Could you check a few things on this model? Use its own coordinates, in mm. A direction names the side the tool comes from. Round coordinates to 2 decimals unless told otherwise and drop trailing zeros. Loops run counter-clockwise (first coordinate to the right, second up) from the corner with the lowest first, then second, coordinate; pieces in that order, holes last. Notation, with made-up numbers: (0.5, 79) -> (39.5, 79) arc R17 ccw to (39.5, 87) -> close; hole circle Ø9 at (-31.5, 66). An arc over 180 degrees is marked (long way). One line per item, written item: value.
from build123d import *

# Parameters (mm, degrees)
BODY_DEPTH                     = 5
BODY_DEPTH_BACK                = 5
SKETCH2_R                      = 0.85
F_1_7MM_THRU_SCREW_HOLES_DEPTH = 15
SCREWHEAD_RELIEF_DEPTH         = 0.5
SKETCH4_R                      = 1.05
F_1_P_PORT_DEPTH               = 5
SKETCH5_R                      = 1.05
F_2_B_PORT_DEPTH               = 5
SKETCH6_R                      = 1.05
F_3_R2_PORT_DEPTH              = 5
SKETCH7_R                      = 1.05
F_4_A_PORT_DEPTH               = 5
SKETCH8_R                      = 1.05
F_5_R1_PORT_DEPTH              = 5
EXTRUDE3_DEPTH                 = 1
FILLET1_R                      = 0.5
SKETCH10_R                     = 0.75
WIRES_2_DEPTH                  = 5


with BuildPart() as part:
    # Sketch1 → Body (new body, two sides)
    with BuildSketch(Plane(origin=(0, 0, 0), x_dir=(0, 0, -1), z_dir=(1, 0, 0))) as body_sk:
        Polygon((0, 0), (-58.6, 0), (-58.6, -14), (-22.5, -14), (-22.5, -19.6), (-4, -19.6), (-4, -14), (0, -14), align=None)
    extrude(amount=BODY_DEPTH)
    extrude(body_sk.sketch, amount=-BODY_DEPTH_BACK)

    # Sketch2 → 1.7mm Thru Screw Holes (cut, through all)
    with BuildSketch(Plane.XZ.offset(14)):
        with Locations(Location((-3.7, 41.9, 0), (0, 0, 270))):  # turned: the seam where the file's is
            Circle(SKETCH2_R)
        with Locations(Location((3.7, 45.5, 0), (0, 0, 270))):  # turned: the seam where the file's is
            Circle(SKETCH2_R)
    extrude(amount=-F_1_7MM_THRU_SCREW_HOLES_DEPTH, mode=Mode.SUBTRACT)

    # Sketch3 → Screwhead Relief (cut)
    with BuildSketch(Plane.XZ.offset(14)):
        with BuildLine():
            Line((-3.7, 43.7), (-5, 43.7))
            Line((-5, 43.7), (-5, 40.1))
            Line((-5, 40.1), (-3.7, 40.1))
            ThreePointArc((-3.7, 40.1), (-1.9, 41.9), (-3.7, 43.7))
        make_face()
        with BuildLine():
            Line((3.7, 47.3), (5, 47.3))
            Line((5, 47.3), (5, 43.7))
            Line((5, 43.7), (3.7, 43.7))
            ThreePointArc((3.7, 43.7), (1.9, 45.5), (3.7, 47.3))
        make_face()
    extrude(amount=-SCREWHEAD_RELIEF_DEPTH, mode=Mode.SUBTRACT)

    # Sketch4 → 1 P _port (cut)
    with BuildSketch(Plane(origin=(0, 0, 0), x_dir=(-1, 0, 0), z_dir=(0, 1, 0))):
        with Locations(Location((0, 43.7, 0), (0, 0, 90))):  # turned: the seam where the file's is
            Circle(SKETCH4_R)
    extrude(amount=-F_1_P_PORT_DEPTH, mode=Mode.SUBTRACT)

    # Sketch5 → 2 B _port (cut)
    with BuildSketch(Plane(origin=(0, 0, 0), x_dir=(-1, 0, 0), z_dir=(0, 1, 0))):
        with Locations(Location((2.5, 47.3, 0), (0, 0, 90))):  # turned: the seam where the file's is
            Circle(SKETCH5_R)
    extrude(amount=-F_2_B_PORT_DEPTH, mode=Mode.SUBTRACT)

    # Sketch6 → 3 R2 _port (cut)
    with BuildSketch(Plane(origin=(0, 0, 0), x_dir=(-1, 0, 0), z_dir=(0, 1, 0))):
        with Locations(Location((0, 50.9, 0), (0, 0, 90))):  # turned: the seam where the file's is
            Circle(SKETCH6_R)
    extrude(amount=-F_3_R2_PORT_DEPTH, mode=Mode.SUBTRACT)

    # Sketch7 → 4 A _port (cut)
    with BuildSketch(Plane(origin=(0, 0, 0), x_dir=(-1, 0, 0), z_dir=(0, 1, 0))):
        with Locations(Location((-2.5, 40.1, 0), (0, 0, 90))):  # turned: the seam where the file's is
            Circle(SKETCH7_R)
    extrude(amount=-F_4_A_PORT_DEPTH, mode=Mode.SUBTRACT)

    # Sketch8 → 5 R1 _port (cut)
    with BuildSketch(Plane(origin=(0, 0, 0), x_dir=(-1, 0, 0), z_dir=(0, 1, 0))):
        with Locations(Location((0, 36.5, 0), (0, 0, 90))):  # turned: the seam where the file's is
            Circle(SKETCH8_R)
    extrude(amount=-F_5_R1_PORT_DEPTH, mode=Mode.SUBTRACT)

    # Sketch9 → Extrude3 (add)
    with BuildSketch(Plane.XZ.offset(19.6)):
        with BuildLine():
            Line((-1.5, 9.5), (1.5, 9.5))
            ThreePointArc((1.5, 9.5), (3.5, 7.5), (1.5, 5.5))
            Line((1.5, 5.5), (-1.5, 5.5))
            ThreePointArc((-1.5, 5.5), (-3.5, 7.5), (-1.5, 9.5))
        make_face()
    extrude(amount=EXTRUDE3_DEPTH)

    # Fillet1
    fillet1_edges = [part.edges().sort_by_distance(p)[0] for p in [
        (-3.5, -20.6, 7.5),
        (0, -20.6, 5.5),
        (3.5, -20.6, 7.5),
        (0, -20.6, 9.5),
    ]]
    fillet(fillet1_edges, radius=FILLET1_R)

    # Sketch10 → Wires 2 (add)
    with BuildSketch(Plane.XZ.offset(20.6)):
        with Locations(Location((-1.5, 7.5, 0), (0, 0, 270))):  # turned: the seam where the file's is
            Circle(SKETCH10_R)
        with Locations(Location((1.5, 7.5, 0), (0, 0, 270))):  # turned: the seam where the file's is
            Circle(SKETCH10_R)
    extrude(amount=WIRES_2_DEPTH)


solid = part.part
(1) I'm going to push flat-ended pins straight in: pin 1 Ø3 at (x, z) = (3, 11) entering from -Y; pin 2 Ø5 at (x, y) = (1, -19.5) entering from +Z; pin 3 Ø3.5 at (x, z) = (0, 43.7) entering from -Y. Where does each tip first touch, or does it pass through?
Recorded:
pin 1: y = -19.6
pin 2: z = 22.5
pin 3: y = -14
(2) If we section it at D-D, the plane x = 0: Please give me the cut outline in (y, z).
Recorded:
outline: (-20.6, 6) arc R0.5 ccw to (-20.1, 5.5) -> (-19.6, 5.5) -> (-19.6, 4) -> (-14, 4) -> (-14, 0) -> (0, 0) -> (0, 35.45) -> (-5, 35.45) -> (-5, 37.55) -> (0, 37.55) -> (0, 42.65) -> (-5, 42.65) -> (-5, 44.75) -> (0, 44.75) -> (0, 49.85) -> (-5, 49.85) -> (-5, 51.95) -> (0, 51.95) -> (0, 58.6) -> (-14, 58.6) -> (-14, 22.5) -> (-19.6, 22.5) -> (-19.6, 9.5) -> (-20.1, 9.5) arc R0.5 ccw to (-20.6, 9) -> close
(3) If I drill on L1, parallel to X at y = -1.1, z = 43.7; L2, parallel to X at y = -5.5, z = 45.5; L3, parallel to Y at x = -0.75, z = 6, over which ranges is the centre line in solid material (lowest first)?
Recorded:
L1: -5 to -1.05, 1.05 to 5
L2: -5 to 2.85, 4.55 to 5
L3: -20.6 to 0
(4) Thinking about a two-plate mould opening in Z: for faces 1 (the face through (-1.5, -25.6, 7.5)), 2 (the face through (2.55, -2.46, 39.05)), 3 (the face through (-3.5, -19.8, 7.5)), which applies, released by +Z, released by -Z, zero draft, split by the parting line, or undercut?
Recorded:
face 1: zero draft
face 2: undercut
face 3: split by the parting line
(5) For faces 4 (the face through (2.78, -13.5, 45.93)), 5 (the face through (-1.47, -23.06, 8.25)), 6 (the face through (3, -5, 40)), 7 (the face through (0, -17, 4)), 8 (the face through (1.5, -25.6, 7.5)), which set-ups out of +Z, -Z, +X, -X, +Y, -Y let a thin tool reach every point of the face, with its end or its side?
Recorded:
face 4: +X, -Y
face 5: -Y
face 6: +Y
face 7: -Z, +X, -X, -Y
face 8: +Z, -Z, +X, -X, -Y
(6) If we section it at C-C, the plane y = -22.5: Please give me the cut outline in (x, z).
Recorded:
outline: circle Ø1.5 at (-1.5, 7.5); circle Ø1.5 at (1.5, 7.5)
(7) If we section it at B-B, the plane z = 36.5: Please give me the cut outline in (x, y), then the cut area to 4 significant figures.
Recorded:
outline: (-5, -14) -> (5, -14) -> (5, 0) -> (1.05, 0) -> (1.05, -5) -> (-1.05, -5) -> (-1.05, 0) -> (-5, 0) -> close
area: 129.5 mm²
(8) If we section it at A-A, the plane y = -3.25: Please give me the cut outline in (x, z), then the cut area to 3 significant figures.
Recorded:
outline: (-5, 0) -> (5, 0) -> (5, 58.6) -> (-5, 58.6) -> close; hole circle Ø1.7 at (-3.7, 41.9); hole circle Ø2.1 at (-2.5, 47.3); hole circle Ø2.1 at (0, 36.5); hole circle Ø2.1 at (0, 43.7); hole circle Ø2.1 at (0, 50.9); hole circle Ø2.1 at (2.5, 40.1); hole circle Ø1.7 at (3.7, 45.5)
area: 564 mm²
